Design review of the part built by this model. Coordinates are the model's own, in mm. Round coordinates to 2 decimals unless told otherwise and drop trailing zeros. Use CSV: the item, a comma, the result in double quotes. Start each with the question number.
Autodesk Inventor part; units mm, degrees
ref_plane "YZ Plane" through (0, 0, 0) normal (1, 0, 0) x (0, 1, 0)
ref_plane "XZ Plane" through (0, 0, 0) normal (0, 1, 0) x (-1, 0, 0)
ref_plane "XY Plane" through (0, 0, 0) normal (0, 0, 1) x (1, 0, 0)
sketch "スケッチ1" plane through (0, 0, 0) normal (0, 0, 1) x (1, 0, 0)
  line L0 (0, 0) -> (-17, 0)
  line L1 (-17, 0) -> (-17, -140)
  line L2 (-17, -140) -> (0, -140)
  line L3 (0, -140) -> (0, 0)
  circle A0 centre (-8.5, -130) radius 1.1
  circle A1 centre (-8.5, -115) radius 1.1
  circle A2 centre (-8.5, -100) radius 1.1
  circle A3 centre (-8.5, -85) radius 1.1
  circle A4 centre (-8.5, -70) radius 1.1
  circle A5 centre (-8.5, -55) radius 1.1
  circle A6 centre (-8.5, -40) radius 1.1
  circle A7 centre (-8.5, -25) radius 1.1
  circle A8 centre (-8.5, -10) radius 1.1
  dimension "d0" = 140
  dimension "d1" = 17
  dimension "d2" = 2.2
  dimension "d3" = 10
  dimension "d4" = 8.5
  dimension "d7" = 15
extrude "押し出し1" add sketch "スケッチ1" along normal blind 0.5
fillet "フィレット1" radius 1 4 edges at (-17, -140, 0.25) (0, -140, 0.25) (0, 0, 0.25) (-17, 0, 0.25)
equation "\"d4\" = 0.5 * d1"
properties part number "Old-sheet"
Q1. The part is to be moulded in two halves that separate along X. For faces 1 (the flat face through (-11, -69, 0.5)), 2 (the cylindrical face through (-7.992, -9.024, 0.246)), say which applies: +X half, -X half, draft (parallel to the pull), parting line (faces both ways), or undercut.
Q2. For L1, parallel to X at y = -100, z = 0.1; L2, parallel to X at y = -129.5, z = 0.3; L3, parallel to Y at x = -0.75, z = 0.2, list the stretches that pass through material, from the lowest coordinate up. Write a range as [from, to].
Q3. Clearance check with a flat-ended pin moving along its axis: pin 1 (1.3 mm diameter, centred on x = -8.5, y = -40, fed in from -Z). State where the tip first meets the part, or that it passes through.
Findings below:
1,face 1,"draft"
1,face 2,"undercut"
2,L1,"x = [-17, -9.6], [-7.4, 0]"
2,L2,"x = [-17, -9.48], [-7.52, 0]"
2,L3,"y = [-139.97, -0.03]"
3,pin 1,"passes through"
